```python
from build123d import *

# Parameters (mm, degrees)
SKETCH1_W           = 322.22857931
SKETCH1_H           = 163.1
BOSS_EXTRUDE1_DEPTH = 6.35
SKETCH2_R           = 10.775
CUT_EXTRUDE1_DEPTH  = 362.210727726
SKETCH4_W           = 322.22857931
SKETCH4_H           = 163.1
BOSS_EXTRUDE3_DEPTH = 3.175


with BuildPart() as part:
    # Sketch1 → Boss-Extrude1 (new body)
    with BuildSketch(Plane.XY):
        with Locations((161.114289655, 81.55)):
            Rectangle(SKETCH1_W, SKETCH1_H)
    extrude(amount=BOSS_EXTRUDE1_DEPTH)

    # Sketch2 → Cut-Extrude1 (cut, through all)
    with BuildSketch(Plane.XY.offset(6.35)):
        with Locations((28.8625, 21.55)):
            Circle(SKETCH2_R)
        with Locations((40.366079306, 45.544994544)):
            Circle(SKETCH2_R)
        with Locations((51.8625, 21.55)):
            Circle(SKETCH2_R)
        with Locations((74.8625, 21.55)):
            Circle(SKETCH2_R)
        with Locations((97.8625, 21.55)):
            Circle(SKETCH2_R)
        with Locations((120.8625, 21.55)):
            Circle(SKETCH2_R)
        with Locations((143.8625, 21.55)):
            Circle(SKETCH2_R)
        with Locations((166.8625, 21.55)):
            Circle(SKETCH2_R)
        with Locations((189.8625, 21.55)):
            Circle(SKETCH2_R)
        with Locations((212.8625, 21.55)):
            Circle(SKETCH2_R)
        with Locations((235.8625, 21.55)):
            Circle(SKETCH2_R)
        with Locations((258.8625, 21.55)):
            Circle(SKETCH2_R)
        with Locations((281.8625, 21.55)):
            Circle(SKETCH2_R)
        with Locations((293.366079306, 45.544994544)):
            Circle(SKETCH2_R)
        with Locations((293.366079306, 93.544994544)):
            Circle(SKETCH2_R)
        with Locations((293.366079306, 141.544994544)):
            Circle(SKETCH2_R)
        with Locations((28.8625, 117.55)):
            Circle(SKETCH2_R)
        with Locations((28.8625, 69.55)):
            Circle(SKETCH2_R)
        with Locations((63.366079306, 45.544994544)):
            Circle(SKETCH2_R)
        with Locations((86.366079306, 45.544994544)):
            Circle(SKETCH2_R)
        with Locations((109.366079306, 45.544994544)):
            Circle(SKETCH2_R)
        with Locations((132.366079306, 45.544994544)):
            Circle(SKETCH2_R)
        with Locations((155.366079306, 45.544994544)):
            Circle(SKETCH2_R)
        with Locations((178.366079306, 45.544994544)):
            Circle(SKETCH2_R)
        with Locations((201.366079306, 45.544994544)):
            Circle(SKETCH2_R)
        with Locations((224.366079306, 45.544994544)):
            Circle(SKETCH2_R)
        with Locations((247.366079306, 45.544994544)):
            Circle(SKETCH2_R)
        with Locations((270.366079306, 45.544994544)):
            Circle(SKETCH2_R)
        with Locations((51.8625, 69.55)):
            Circle(SKETCH2_R)
        with Locations((74.8625, 69.55)):
            Circle(SKETCH2_R)
        with Locations((97.8625, 69.55)):
            Circle(SKETCH2_R)
        with Locations((120.8625, 69.55)):
            Circle(SKETCH2_R)
        with Locations((143.8625, 69.55)):
            Circle(SKETCH2_R)
        with Locations((166.8625, 69.55)):
            Circle(SKETCH2_R)
        with Locations((189.8625, 69.55)):
            Circle(SKETCH2_R)
        with Locations((212.8625, 69.55)):
            Circle(SKETCH2_R)
        with Locations((235.8625, 69.55)):
            Circle(SKETCH2_R)
        with Locations((258.8625, 69.55)):
            Circle(SKETCH2_R)
        with Locations((281.8625, 69.55)):
            Circle(SKETCH2_R)
        with Locations((51.8625, 117.55)):
            Circle(SKETCH2_R)
        with Locations((74.8625, 117.55)):
            Circle(SKETCH2_R)
        with Locations((97.8625, 117.55)):
            Circle(SKETCH2_R)
        with Locations((120.8625, 117.55)):
            Circle(SKETCH2_R)
        with Locations((143.8625, 117.55)):
            Circle(SKETCH2_R)
        with Locations((166.8625, 117.55)):
            Circle(SKETCH2_R)
        with Locations((189.8625, 117.55)):
            Circle(SKETCH2_R)
        with Locations((212.8625, 117.55)):
            Circle(SKETCH2_R)
        with Locations((235.8625, 117.55)):
            Circle(SKETCH2_R)
        with Locations((258.8625, 117.55)):
            Circle(SKETCH2_R)
        with Locations((281.8625, 117.55)):
            Circle(SKETCH2_R)
        with Locations((40.366079306, 93.544994544)):
            Circle(SKETCH2_R)
        with Locations((63.366079306, 93.544994544)):
            Circle(SKETCH2_R)
        with Locations((86.366079306, 93.544994544)):
            Circle(SKETCH2_R)
        with Locations((109.366079306, 93.544994544)):
            Circle(SKETCH2_R)
        with Locations((132.366079306, 93.544994544)):
            Circle(SKETCH2_R)
        with Locations((155.366079306, 93.544994544)):
            Circle(SKETCH2_R)
        with Locations((178.366079306, 93.544994544)):
            Circle(SKETCH2_R)
        with Locations((201.366079306, 93.544994544)):
            Circle(SKETCH2_R)
        with Locations((224.366079306, 93.544994544)):
            Circle(SKETCH2_R)
        with Locations((247.366079306, 93.544994544)):
            Circle(SKETCH2_R)
        with Locations((270.366079306, 93.544994544)):
            Circle(SKETCH2_R)
        with Locations((40.366079306, 141.544994544)):
            Circle(SKETCH2_R)
        with Locations((63.366079306, 141.544994544)):
            Circle(SKETCH2_R)
        with Locations((86.366079306, 141.544994544)):
            Circle(SKETCH2_R)
        with Locations((109.366079306, 141.544994544)):
            Circle(SKETCH2_R)
        with Locations((132.366079306, 141.544994544)):
            Circle(SKETCH2_R)
        with Locations((155.366079306, 141.544994544)):
            Circle(SKETCH2_R)
        with Locations((178.366079306, 141.544994544)):
            Circle(SKETCH2_R)
        with Locations((201.366079306, 141.544994544)):
            Circle(SKETCH2_R)
        with Locations((224.366079306, 141.544994544)):
            Circle(SKETCH2_R)
        with Locations((247.366079306, 141.544994544)):
            Circle(SKETCH2_R)
        with Locations((270.366079306, 141.544994544)):
            Circle(SKETCH2_R)
    extrude(amount=-CUT_EXTRUDE1_DEPTH, mode=Mode.SUBTRACT)

    # Sketch4 → Boss-Extrude3 (add)
    with BuildSketch(Plane(origin=(0, 0, 0), x_dir=(-1, 0, 0), z_dir=(0, 0, -1))):
        with Locations((-161.114289655, 81.55)):
            Rectangle(SKETCH4_W, SKETCH4_H)
    extrude(amount=BOSS_EXTRUDE3_DEPTH)


solid = part.part
```
Design review of the part built by this model. Coordinates are the model's own, in mm. Round coordinates to 2 decimals unless told otherwise and drop trailing zeros. One line per question, with ' | ' between items.
Item 1: Draft analysis for pull direction Y (two halves, no side actions). For faces 1 (the face through (123, 83, 6.35)), 2 (the face through (163, 163.1, 2)), 3 (the face through (271, 46, 0)), state which applies: +Y half, -Y half, draft (parallel to the pull), parting line (faces both ways), or undercut.
Checks:
face 1: draft | face 2: +Y half | face 3: undercut
Item 2: Take a section at A-A, the plane z = 4.5. Give the number of separate pieces and of enclosed holes in the cut face, then the cut area to 3 significant figures.
Checks:
separate pieces: 1 | enclosed holes: 72 | area: 26,300 mm²
Item 3: For P1, Ø19.5, axis at x = 189.86, y = 117.55, coming from the +Z side; P2, Ø6, axis at x = 168.5, y = 96, coming from the +Z side, all flat-tipped, find the tip position at first contact; note any pin that passes through.
Checks:
P1: z = 0 | P2: z = 6.35
Item 4: Wall thickness on line 1 (Z direction, x = 60, y = 100) (3 decimals): over which ranges is the line inside the solid? List them lowest first. Write a range as [from, to].
Checks:
line 1: [-3.175, 0]
